Build history of the part. All positions in model axes, mm. Face numbers are marked on the shaded views. A direction names the side the tool comes from. Round coordinates to 2 decimals unless told otherwise and drop trailing zeros. Write each loop counter-clockwise with the first axis right and the second up, starting at its lowest first coordinate (ties: lowest second). Pieces come first, ordered by that corner, then holes. Notation, with made-up numbers: (12.25, 54) - (67.25, 54) arc R31 ccw to (67.25, 80) - close; hole circle Ø6 at (42.5, -29). An arc over 180 degrees is marked (long way). Write each question's results on one line, items separated by ' | '.
from build123d import *

# Parameters (mm, degrees)
SKETCH1_R           = 1.6
BOSS_EXTRUDE1_DEPTH = 4
SKETCH1_4_R         = 4
SKETCH1_4_R_2       = 1.6
BOSS_EXTRUDE2_DEPTH = 18
SKETCH3_R           = 3.6
SKETCH3_R_2         = 1.6
BOSS_EXTRUDE3_DEPTH = 0.5
FILLET1_R           = 2


with BuildPart() as part:
    # Sketch1 → Boss-Extrude1 (new body)
    with BuildSketch(Plane.XY):
        with BuildLine():
            Line((-36, 15.5), (-6, -24.5))
            ThreePointArc((-6, -24.5), (0, -27.5), (6, -24.5))
            Line((6, -24.5), (36, 15.5))
            ThreePointArc((36, 15.5), (36.708203932, 23.354101966), (30, 27.5))
            Line((30, 27.5), (-30, 27.5))
            ThreePointArc((-30, 27.5), (-36.708203932, 23.354101966), (-36, 15.5))
        make_face()
        with Locations((-30, 20)):
            Circle(SKETCH1_R, mode=Mode.SUBTRACT)
        with Locations((30, 20)):
            Circle(SKETCH1_R, mode=Mode.SUBTRACT)
        with Locations((0, 20)):
            Circle(SKETCH1_R, mode=Mode.SUBTRACT)
        with Locations((0, -20)):
            Circle(SKETCH1_R, mode=Mode.SUBTRACT)
    extrude(amount=BOSS_EXTRUDE1_DEPTH)

    # Sketch1<4> → Boss-Extrude2 (add)
    with BuildSketch(Plane.XY):
        with Locations((0, 20)):
            Circle(SKETCH1_4_R)
        with Locations((0, 20)):
            Circle(SKETCH1_4_R_2, mode=Mode.SUBTRACT)
        with Locations((0, -20)):
            Circle(SKETCH1_4_R)
        with Locations((0, -20)):
            Circle(SKETCH1_4_R_2, mode=Mode.SUBTRACT)
    extrude(amount=-BOSS_EXTRUDE2_DEPTH)

    # Sketch3 → Boss-Extrude3 (add)
    with BuildSketch(Plane(origin=(0, 0, 0), x_dir=(-1, 0, 0), z_dir=(0, 0, -1))):
        with Locations((-30, 20)):
            Circle(SKETCH3_R)
        with Locations((-30, 20)):
            Circle(SKETCH3_R_2, mode=Mode.SUBTRACT)
        with Locations((30, 20)):
            Circle(SKETCH3_R)
        with Locations((30, 20)):
            Circle(SKETCH3_R_2, mode=Mode.SUBTRACT)
    extrude(amount=BOSS_EXTRUDE3_DEPTH)

    # Fillet1
    fillet1_edges = [part.edges().sort_by_distance(p)[0] for p in [
        (-4, 20, 0),
        (-4, -20, 0),
    ]]
    fillet(fillet1_edges, radius=FILLET1_R)


solid = part.part
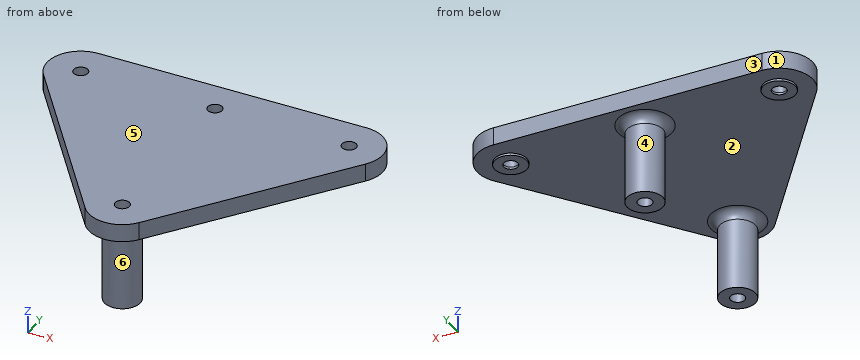
(1) Drill centre lines: probe 1 along Y at (x, z) = (0, 2.5); probe 2 along Y at (x, z) = (0, -3.75); probe 3 along Y at (x, z) = (-30, -0.1). Where is each one in solid material? Low to high. Write a range as [from, to].
Worked answers:
probe 1: y = [-27.5, -21.6], [-18.4, 18.4], [21.6, 27.5] | probe 2: y = [-24, -21.6], [-18.4, -16], [16, 18.4], [21.6, 24] | probe 3: y = [16.4, 18.4], [21.6, 23.6]
(2) Slice it at B-B, the plane y = 20. State how many separate pieces and enclosed holes the cut face has, and give its area (3 significant figures).
Worked answers:
separate pieces: 4 | enclosed holes: 0 | area: 354 mm2
(3) Two-plate mould, pull along Y, no slides. Class the marked faces 3, 4, 5 and 6: released by +Y, released by -Y, zero draft, split by the parting line, or undercut.
Worked answers:
face 3: released by +Y | face 4: undercut | face 5: zero draft | face 6: undercut
(4) Slice it at C-C, the plane z = -3.5. Write the cut outline in (x, y).
Worked answers:
outline: circle Ø8 at (0, -20); circle Ø8 at (0, 20); hole circle Ø3.2 at (0, -20); hole circle Ø3.2 at (0, 20)
(5) Tool access for the marked faces 1 and 2: list every direction of +Z, -Z, +X, -X, +Y, -Y with a clear straight run to the whole face (end or side of a thin tool).
Worked answers:
face 1: +Z, -Z, -X | face 2: -Z
(6) Slice it at A-A, the plane x = 0. Write the cut outline in (y, z).
Worked answers:
outline: (-27.5, 0) - (-26, 0) arc R2 cw to (-24, -2) - (-24, -18) - (-21.6, -18) - (-21.6, 4) - (-27.5, 4) - close; (-18.4, -18) - (-16, -18) - (-16, -2) arc R2 cw to (-14, 0) - (14, 0) arc R2 cw to (16, -2) - (16, -18) - (18.4, -18) - (18.4, 4) - (-18.4, 4) - close; (21.6, -18) - (24, -18) - (24, -2) arc R2 cw to (26, 0) - (27.5, 0) - (27.5, 4) - (21.6, 4) - close
(7) Slice it at D-D, the plane y = -20. Write the cut outline in (x, z) (3 decimals).
Worked answers:
outline: (-9.375, 0) - (-6, 0) arc R2 cw to (-4, -2) - (-4, -18) - (-1.6, -18) - (-1.6, 4) - (-9.375, 4) - close; (1.6, -18) - (4, -18) - (4, -2) arc R2 cw to (6, 0) - (9.375, 0) - (9.375, 4) - (1.6, 4) - close
(8) Flat gauge pins, fed straight in: pin 1 Ø2 at (x, y) = (-30.5, 18) entering from -Z; pin 2 Ø6 at (y, z) = (4.5, 1) entering from +X; pin 3 Ø2 at (y, z) = (-20, -13.5) entering from -X. Where does each tip first touch, or does it go through?
Worked answers:
pin 1: stops at z = -0.5 | pin 2: stops at x = 30 | pin 3: stops at x = -4
